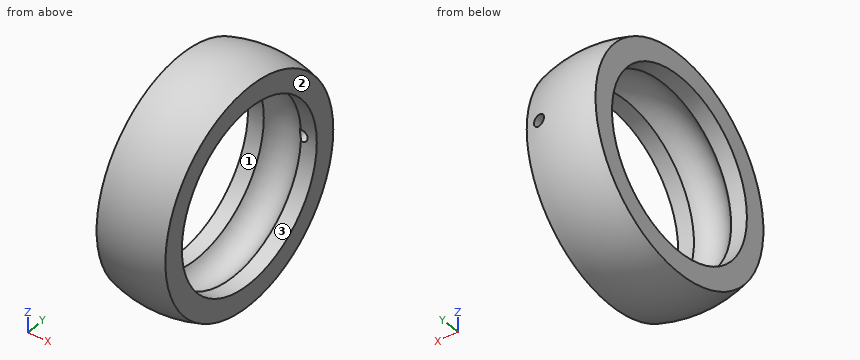
Solid Edge part; units mm, degrees
sketch "Sketch1" plane through (0, 0, 0) normal (0, 0, 1) x (1, 0, 0)
  line L0 (5.5, 19.0788) -> (5.5, 15.3333)
  line L1 (5.5, 15.3333) -> (8.2511, 15.3333)
  arc A0 (8.2511, 15.3333) -> (14.7489, 15.3333) centre (11.5, 13) cw
  line L2 (14.7489, 15.3333) -> (17.5, 15.3333)
  line L3 (17.5, 15.3333) -> (17.5, 19.0788)
  arc A1 (17.5, 19.0788) -> (5.5, 19.0788) centre (11.5, 0) ccw
revolve "RevolvedProtrusion1" add sketch "Sketch1" angle 360 about axis through (17.5, 0, 0) along (-1, 0, 0)
sketch "Sketch2" plane through (0, 0, 0) normal (0, -1, 0) x (1, 0, 0)
  circle A0 centre (14.9, 0) radius 1
extrude "Cutout1" cut sketch "Sketch2" against normal blind 40
properties part number "UCP201 GB/T7810-1995_PART1"
Read the model definition and answer for the solid it produces. Units are mm, in the model's axes. Face numbers are marked on the shaded views. Coordinates: 2 decimals unless noted, no trailing zeros. Loops run counter-clockwise (first coordinate to the right, second up) from the corner with the lowest first, then second, coordinate; pieces in that order, holes last.
Q1. Consider probe 1 along Y at (x, z) = (11.75, -5.5); probe 2 along Z at (x, y) = (14, 16.5); probe 3 along Y at (x, z) = (6, -14). Determine where each line is inside the solid, lowest interval first.
Q2. The part is cut by section B-B on z = 0. Write down the section's boundary in (x, y).
Q3. The part is cut by section A-A on y = 0. Write down the section's boundary in (x, z).
Q4. The mould has two halves that part along Y. Classify the marked faces 1, 2 and 3: +Y half, -Y half, draft (parallel to the pull), parting line (faces both ways), or undercut.
Q5. Each of these flat-tipped pins is pushed along its axis until it touches: pin 1 Ø2 at (x, y) = (15.5, -12) entering from -Z; pin 2 Ø1 at (x, z) = (12, 6) entering from +Y; pin 3 Ø1.6 at (x, z) = (14.9, 0) entering from +Y. Where does it stop, or does it pass through?
Results below:
1. probe 1: y = -19.23 to -16.08, 16.08 to 19.23
1. probe 2: z = -11.02 to -0.44, 0.44 to 11.02
1. probe 3: y = -13.18 to -6.25, 6.25 to 13.18
2. outline: (5.5, -19.08) arc R20 ccw to (17.5, -19.08) - (17.5, -15.33) - (14.75, -15.33) arc R4 cw to (8.25, -15.33) - (5.5, -15.33) - close; (5.5, 15.33) - (8.25, 15.33) arc R4 cw to (13.9, 16.2) - (13.9, 19.86) arc R20 ccw to (5.5, 19.08) - close; (15.9, 15.33) - (17.5, 15.33) - (17.5, 19.08) arc R20 ccw to (15.9, 19.51) - close
3. outline: (5.5, -19.08) arc R20 ccw to (17.5, -19.08) - (17.5, -15.33) - (14.75, -15.33) arc R4 cw to (8.25, -15.33) - (5.5, -15.33) - close; (5.5, 15.33) - (8.25, 15.33) arc R4 cw to (14.75, 15.33) - (17.5, 15.33) - (17.5, 19.08) arc R20 ccw to (5.5, 19.08) - close
4. face 1: undercut
4. face 2: draft
4. face 3: undercut
5. pin 1: stops at z = -16.26
5. pin 2: stops at y = 19.22
5. pin 3: stops at y = -15.31
